from build123d import *

# Parameters (mm, degrees)
SKETCH1_R           = 3.5
SKETCH1_R_2         = 2.1
BOSS_EXTRUDE1_DEPTH = 4.7
BOSS_EXTRUDE2_START = -2
SKETCH3_R           = 2.1
SKETCH3_R_2         = 1.4
BOSS_EXTRUDE2_DEPTH = 1
BOSS_EXTRUDE3_START = -2.7
BOSS_EXTRUDE3_DEPTH = 2.2
CUT_EXTRUDE1_REACH  = 20.946
SKETCH5_R           = 1.15


with BuildPart() as part:
    # Sketch1 → Boss-Extrude1 (new body)
    with BuildSketch(Plane(origin=(0, 0, 0), x_dir=(1, 0, 0), z_dir=(0, 1, 0))):
        with Locations(Location((0, 0, 0), (0, 0, 270))):
            Circle(SKETCH1_R)
        with Locations(Location((0, 0, 0), (0, 0, 270))):
            Circle(SKETCH1_R_2, mode=Mode.SUBTRACT)
    extrude(amount=BOSS_EXTRUDE1_DEPTH)

    # Sketch3 → Boss-Extrude2 (add)
    with BuildSketch(Plane(origin=(0, 4.7, 0), x_dir=(1, 0, 0), z_dir=(0, 1, 0)).offset(BOSS_EXTRUDE2_START)):
        with Locations(Location((0, 0, 0), (0, 0, 270))):
            Circle(SKETCH3_R)
        with Locations(Location((0, 0, 0), (0, 0, 270))):
            Circle(SKETCH3_R_2, mode=Mode.SUBTRACT)
    extrude(amount=BOSS_EXTRUDE2_DEPTH)

    # Sketch4 → Boss-Extrude3 (add)
    with BuildSketch(Plane(origin=(0, 4.7, 0), x_dir=(1, 0, 0), z_dir=(0, 1, 0)).offset(BOSS_EXTRUDE3_START)):
        with BuildLine():
            Line((-0.335083385, 3.483922951), (-16.376689314, 1.941042787))
            ThreePointArc((-16.376689314, 1.941042787), (-18.14, 0), (-16.376689314, -1.941042787))
            Line((-16.376689314, -1.941042787), (-0.335083385, -3.483922951))
            ThreePointArc((-0.335083385, -3.483922951), (-3.5, 0), (-0.335083385, 3.483922951))
        make_face()
    extrude(amount=BOSS_EXTRUDE3_DEPTH)

    # Sketch5 → Cut-Extrude1 (cut, up to next)
    with BuildSketch(Plane(origin=(0, 4.2, 0), x_dir=(1, 0, 0), z_dir=(0, 1, 0)), mode=Mode.PRIVATE) as cut_extrude1_sk1:
        with Locations(Location((-14.35, 0, 0), (0, 0, 270))):
            Circle(SKETCH5_R)
    cut_extrude1_tool1 = extrude(cut_extrude1_sk1.sketch, amount=-CUT_EXTRUDE1_REACH, mode=Mode.PRIVATE) & part.part
    # Sketch5 → Cut-Extrude1 (cut, up to next)
    with BuildSketch(Plane(origin=(0, 4.2, 0), x_dir=(1, 0, 0), z_dir=(0, 1, 0)), mode=Mode.PRIVATE) as cut_extrude1_sk2:
        with Locations(Location((-6.25, 0, 0), (0, 0, 270))):
            Circle(SKETCH5_R)
    cut_extrude1_tool2 = extrude(cut_extrude1_sk2.sketch, amount=-CUT_EXTRUDE1_REACH, mode=Mode.PRIVATE) & part.part
    add(cut_extrude1_tool1.solids().sort_by_distance((-14.35, 4.2, 0))[0], mode=Mode.SUBTRACT)
    add(cut_extrude1_tool2.solids().sort_by_distance((-6.25, 4.2, 0))[0], mode=Mode.SUBTRACT)


solid = part.part
Build history of the part. All positions in model axes, mm. A direction names the side the tool comes from. Round coordinates to 2 decimals unless told otherwise and drop trailing zeros. Write each loop counter-clockwise with the first axis right and the second up, starting at its lowest first coordinate (ties: lowest second). Pieces come first, ordered by that corner, then holes. Notation, with made-up numbers: (41, 42.5) - (45, 42.5) arc R21 cw to (45, 80.5) - close; hole circle Ø8 at (32, 13.25). An arc over 180 degrees is marked (long way). Use CSV: the item, a comma, the result in double quotes.
(1) Wall check: line 1 (X direction, y = 3.3, z = 0); line 2 (X direction, y = 4.1, z = 0); line 3 (X direction, y = 0.3, z = 0). Give the ranges that are in metal, low to high.
Response:
line 1,"-18.14 to -15.5, -13.2 to -7.4, -5.1 to -1.4, 1.4 to 3.5"
line 2,"-18.14 to -15.5, -13.2 to -7.4, -5.1 to -2.1, 2.1 to 3.5"
line 3,"-3.5 to -2.1, 2.1 to 3.5"
(2) Band-saw the part on B-B (z = 0). Write the cut outline in (x, y).
Response:
outline,"(-18.14, 2) - (-15.5, 2) - (-15.5, 4.2) - (-18.14, 4.2) - close; (-13.2, 2) - (-7.4, 2) - (-7.4, 4.2) - (-13.2, 4.2) - close; (-5.1, 2) - (-3.5, 2) - (-3.5, 0) - (-2.1, 0) - (-2.1, 2.7) - (-1.4, 2.7) - (-1.4, 3.7) - (-2.1, 3.7) - (-2.1, 4.7) - (-3.5, 4.7) - (-3.5, 4.2) - (-5.1, 4.2) - close; (1.4, 2.7) - (2.1, 2.7) - (2.1, 0) - (3.5, 0) - (3.5, 4.7) - (2.1, 4.7) - (2.1, 3.7) - (1.4, 3.7) - close"
(3) Mould opens along Z. For faces 3 (the cylindrical face through (0.631, 1.331, 2.003)), 4 (the flat face through (-8.244, 3.085, -2.723)), 5 (the cylindrical face through (0.06, 3.19, -1.4)), 6 (the flat face through (-8.5, 3.1, 2.7)) say: pulls with the +Z half, pulls with the -Z half, needs draft (parallel to the pull), parting line crosses it, or undercut.
Response:
face 3,"undercut"
face 4,"pulls with the -Z half"
face 5,"undercut"
face 6,"pulls with the +Z half"
(4) Band-saw the part on D-D (x = -13.75). Write the cut outline in (y, z).
Response:
outline,"(2, -2.19) - (4.2, -2.19) - (4.2, -0.98) - (2, -0.98) - close; (2, 0.98) - (4.2, 0.98) - (4.2, 2.19) - (2, 2.19) - close"
(5) Pin check, flat tips, straight feed: P1, Ø3.5, axis at x = 0, z = 0, coming from the -Y side; P2, Ø2, axis at x = -5, z = 0.5, coming from the -Y side; P3, Ø1.3, axis at x = 0, z = 0, coming from the -Y side. Stop position of each tip, or through.
Response:
P1,"y = 2.7"
P2,"y = 2"
P3,"through"
(6) Band-saw the part on C-C (y = 3.35). Write the cut outline in (x, z), plus the area to 3 significant figures.
Response:
outline,"(-16.38, -1.94) - (-0.34, -3.48) arc R3.5 ccw (long way) to (-0.34, 3.48) - (-16.38, 1.94) arc R1.95 ccw to start; hole circle Ø2.3 at (-14.35, 0); hole circle Ø2.3 at (-6.25, 0); hole circle Ø2.8 at (0, 0)"
area,"99.4 mm²"
(7) 3-axis set-ups, long thin cutter, end or side, ignore diameter. For faces 1 (the flat face through (-2, 4.7, 2)), 2 (the cylindrical face through (0.631, 4.193, 2.003)): which of +Z, -Z, +X, -X, +Y, -Y reach the whole face in a straight line?
Response:
face 1,"+Z, -Z, +X, -X, +Y"
face 2,"+Y"
(8) Band-saw the part on A-A (x = 0). Write the cut outline in (y, z), plus the area to 3 significant figures.
Response:
outline,"(0, -3.5) - (4.7, -3.5) - (4.7, -2.1) - (3.7, -2.1) - (3.7, -1.4) - (2.7, -1.4) - (2.7, -2.1) - (0, -2.1) - close; (0, 2.1) - (2.7, 2.1) - (2.7, 1.4) - (3.7, 1.4) - (3.7, 2.1) - (4.7, 2.1) - (4.7, 3.5) - (0, 3.5) - close"
area,"14.6 mm²"
